Check sheet for the modelled part. Datum: model origin and axes. Units: mm. Face numbers are marked on the shaded views. A direction names the side the tool comes from. Coordinates: 2 decimals unless noted, no trailing zeros. Write each loop counter-clockwise with the first axis right and the second up, starting at its lowest first coordinate (ties: lowest second). Pieces come first, ordered by that corner, then holes. Notation, with made-up numbers: M 78.25,-35.5 L 134.25,-35.5 A21 cw 134.25,-12.5 Z; hole C 12.25,23.25 d5. An arc over 180 degrees is marked long. Answer as CSV lines item,"result". Start each with the question number.
Q1. Mould release check, pull along X, two halves, no side actions. Record for the marked faces 4, 5, 6 and 7: pulls with the +X half, pulls with the -X half, needs draft (parallel to the pull), parting line crosses it, or undercut.
Q2. Sectioned sample at C-C, the plane y = -6. Record the cut outline in (x, z), then the cut area to 3 significant figures.
Q3. Thickness scan on line 1 along Y through (x, z) = (-16, -11); line 2 along Y through (x, z) = (0.5, 1.5); line 3 along X through (y, z) = (-9.5, 1). Record the ranges inside material, lowest first. Write a range as from..to.
Q4. Sectioned sample at D-D, the plane x = 0. Record the cut outline in (y, z).
Q5. Depth check by flat-ended pin: pin 1 Ø1 at (x, z) = (-9, -10.5) entering from -Y; pin 2 Ø9 at (x, z) = (-22, -0.5) entering from +Y; pin 3 Ø16 at (x, z) = (-15, -0.5) entering from -Y. Enter the tip coordinate at first touch or a pass-through.
Q6. Access from +Z, -Z, +X, -X, +Y, -Y to the whole of each face (thin tool, end or side, straight path). Record for the marked faces 1, 2 and 3.
Q7. Sectioned sample at B-B, the plane z = 11.5. Record the cut outline in (x, y).
Q8. Sectioned sample at A-A, the plane x = -10.5. Record the cut outline in (y, z).
Autodesk Inventor part; units mm, degrees
ref_plane "Work Plane1" through (0, 8, 0) normal (0, 1, 0) x (-1, 0, 0)
ref_plane "Length_WKP" through (0, -35, 0) normal (0, 1, 0) x (-1, 0, 0)
ref_plane "Work Plane3" through (0, -15, 0) normal (0, 1, 0) x (-1, 0, 0)
sketch "Sketch1" plane through (0, 0, 0) normal (0, 0, 1) x (1, 0, 0)
  circle A0 centre (0, 0) radius 7.5
  circle A1 centre (0, 0) radius 9.5
  dimension "d0" = 15
  dimension "d1" = 2
extrude "Extrusion1" add sketch "Sketch1" along normal mid plane 30
sketch "Sketch3" plane through (0, 0, 0) normal (0, 0, 1) x (1, 0, 0)
  circle A0 centre (0, 0) radius 9.5
  line L0 (-27.5, 2.5) -> (-27.5, -2.5)
  line L1 (-27.5, 2.5) -> (-9.1652, 2.5)
  line L2 (-27.5, -2.5) -> (-9.1652, -2.5)
  line L3 (27.5, 2.5) -> (27.5, -2.5)
  line L4 (27.5, 2.5) -> (9.1652, 2.5)
  line L5 (27.5, -2.5) -> (9.1652, -2.5)
  point P0 (-27.5, 0)
  point P1 (27.5, 0)
  dimension "d4" = 5
  dimension "d6" = 5
  dimension "d22" = 27.5
  dimension "d23" = 27.5
extrude "Extrusion2" add sketch "Sketch3" along normal mid plane 30 contours A0 L4 L3 L5 | A0 L2 L0 L1
sketch "Sketch10" plane through (0, 0, 0) normal (0, 0, 1) x (1, 0, 0)
  line L0 (-27.5, -2.5) -> (-27.5, 2.5)
  line L1 (27.5, 2.5) -> (27.5, -2.5)
  line L2 (-27.5, -0.5) -> (27.5, -0.5)
  line L3 (27.5, -0.5) -> (27.5, 0.5)
  line L4 (27.5, 0.5) -> (-27.5, 0.5)
  line L5 (-27.5, 0.5) -> (-27.5, -0.5)
  line L6 (27.5, -2.5) -> (9.1652, -2.5)
  line L7 (9.1652, 2.5) -> (27.5, 2.5)
  point P0 (0, 0)
  dimension "d28" = 2
  dimension "d29" = 2
extrude "Extrusion7" cut sketch "Sketch10" along normal through all both and the other way through all
sketch "Sketch4" plane through (-27.5, -2.5, -15) normal (0, -1, 0) x (1, 0, 0)
  line L0 (18.3348, 30) -> (0, 30)
  line L1 (0, 0) -> (0, 30)
  line L2 (55, 30) -> (36.6652, 30)
  line L3 (36.6652, 0) -> (36.6652, 30)
  line L4 (36.6652, 0) -> (55, 0)
  line L5 (55, 0) -> (55, 30)
  circle A0 centre (9.1674, 15) radius 3
  circle A1 centre (45.8326, 15) radius 3
  point P0 (0, 15)
  point P1 (9.1674, 30)
  point P2 (45.8326, 30)
  point P3 (55, 15)
  dimension "d10" = 6
  dimension "d11" = 6
extrude "Extrusion3" add sketch "Sketch4" along normal mid plane 15 contours A0 | A1
ref_plane "Work Plane1" through (0, 8, 0) normal (0, 1, 0) x (-1, 0, 0)
sketch "Sketch6" plane through (0, 8, 0) normal (0, 1, 0) x (-1, 0, 0)
  circle A0 centre (-18.3326, 0) radius 3
  circle A1 centre (18.3326, 0) radius 3
  line L0 (-19.7333, -5.601) -> (-23.8836, -1.5874)
  line L1 (-23.8836, -1.5874) -> (-22.4828, 4.0136)
  line L2 (-22.4828, 4.0136) -> (-16.9318, 5.601)
  line L3 (-16.9318, 5.601) -> (-12.7816, 1.5874)
  line L4 (-12.7816, 1.5874) -> (-14.1824, -4.0136)
  line L5 (-14.1824, -4.0136) -> (-19.7333, -5.601)
  line L6 (20.6316, -5.296) -> (14.8956, -4.639)
  line L7 (14.8956, -4.639) -> (12.5966, 0.657)
  line L8 (12.5966, 0.657) -> (16.0335, 5.296)
  line L9 (16.0335, 5.296) -> (21.7695, 4.639)
  line L10 (21.7695, 4.639) -> (24.0686, -0.657)
  line L11 (24.0686, -0.657) -> (20.6316, -5.296)
  dimension "d15" = 10
extrude "Extrusion4" add sketch "Sketch6" against normal up to surface (5.5 mm away) contours A0 | A1 | L0 L1 L2 L3 L4 L5 | L6 L7 L8 L9 L10 L11
ref_plane "Length_WKP" through (0, -35, 0) normal (0, 1, 0) x (-1, 0, 0)
sketch "Sketch8" plane through (0, -35, 0) normal (0, 1, 0) x (-1, 0, 0)
  line L0 (-38.5, 0) -> (38.5, 0)
  line L1 (0, -21) -> (0, 21)
  circle A0 centre (0, 0) radius 5
  dimension "d19" = 10
extrude "Extrusion5" add sketch "Sketch8" along normal up to next
ref_plane "Work Plane3" through (0, -15, 0) normal (0, 1, 0) x (-1, 0, 0)
sketch "Sketch9" plane through (0, -15, 0) normal (0, 1, 0) x (-1, 0, 0)
  circle A0 centre (0, 0) radius 5
  circle A1 centre (0, 0) radius 9
  dimension "d25" = 4
extrude "Extrusion6" add sketch "Sketch9" along normal up to next
mirror "Mirror1" about plane through (0, 0, 0) normal (0, 1, 0) of "Extrusion4"
equation "\"d0\" = dia"
equation "\"d2\" = Bredde"
equation "\"d8\" = Bredde"
equation "\"d29\" = d28"
equation "\"d11\" = d10"
equation "\"dia\" = 15"
equation "\"Bredde\" = 30"
properties part number "Pipe Clamp - Ø25" material "Stainless Steel"
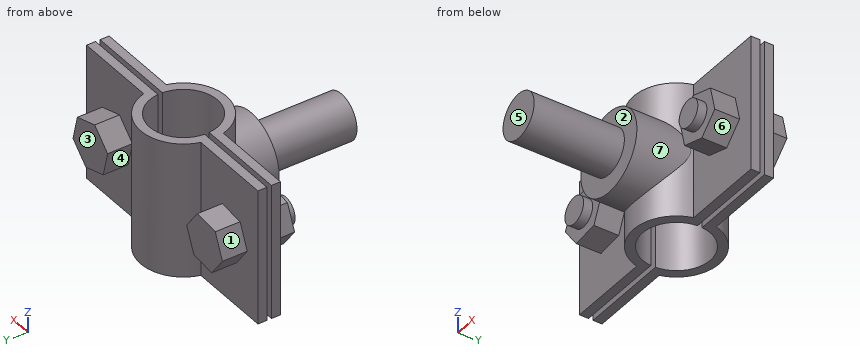
Output:
1,face 4,"undercut"
1,face 5,"needs draft"
1,face 6,"pulls with the +X half"
1,face 7,"undercut"
2,outline,"M -24.07,-0.66 L -20.63,-5.3 L -14.9,-4.64 L -12.6,0.66 L -16.03,5.3 L -21.77,4.64 Z; M -7.37,-15 L -4.5,-15 L -4.5,15 L -7.37,15 L -7.37,5.17 A9 ccw -7.37,-5.17 Z; M 4.5,-15 L 7.37,-15 L 7.37,-5.17 A9 ccw 7.37,5.17 L 7.37,15 L 4.5,15 Z; M 12.78,1.59 L 14.18,-4.01 L 19.73,-5.6 L 23.88,-1.59 L 22.48,4.01 L 16.93,5.6 Z"
2,area,"368 mm^2"
3,line 1,"y = -2.5..-0.5, 0.5..2.5"
3,line 2,"y = -35..-7.48, 7.48..9.49"
3,line 3,"x = -21.16..-15.5, -8.94..8.94, 15.5..21.16"
4,outline,"M -35,-5 L -15,-5 L -15,-9 L -9.5,-9 L -9.5,-15 L -7.5,-15 L -7.5,15 L -9.5,15 L -9.5,9 L -15,9 L -15,5 L -35,5 Z; M 7.5,-15 L 9.5,-15 L 9.5,15 L 7.5,15 Z"
5,pin 1,"stops at y = -4.24"
5,pin 2,"stops at y = 8"
5,pin 3,"stops at y = -15"
6,face 1,"+Z, -X, +Y"
6,face 2,"-Y"
6,face 3,"+Z, -Z, +X, +Y"
7,outline,"M -27.5,-2.5 L -9.17,-2.5 A9.5 ccw 9.17,-2.5 L 27.5,-2.5 L 27.5,-0.5 L 7.48,-0.5 A7.5 cw -7.48,-0.5 L -27.5,-0.5 Z; M -27.5,0.5 L -7.48,0.5 A7.5 cw 7.48,0.5 L 27.5,0.5 L 27.5,2.5 L 9.17,2.5 A9.5 ccw -9.17,2.5 L -27.5,2.5 Z"
8,outline,"M -2.5,-15 L -0.5,-15 L -0.5,15 L -2.5,15 Z; M 0.5,-15 L 2.5,-15 L 2.5,15 L 0.5,15 Z"
